Geometry check sheet. Reference: drawing and pictorial views, mm from the part's lowest x, y, z. A direction names the side the tool comes from. Coordinates: 2 decimals unless noted, no trailing zeros. Order: outer loops, then holes, each group sorted by start corner. A loop starts at its lowest first (then second) coordinate and runs counter-clockwise, first axis right, second up. Notation, with made-up numbers: M 29.5,50 L 59.5,50 A21 ccw 59.5,67 Z; hole C 48,-1 d7. An arc over 180 degrees is marked long. Return JSON: item names as keys, results as strings.
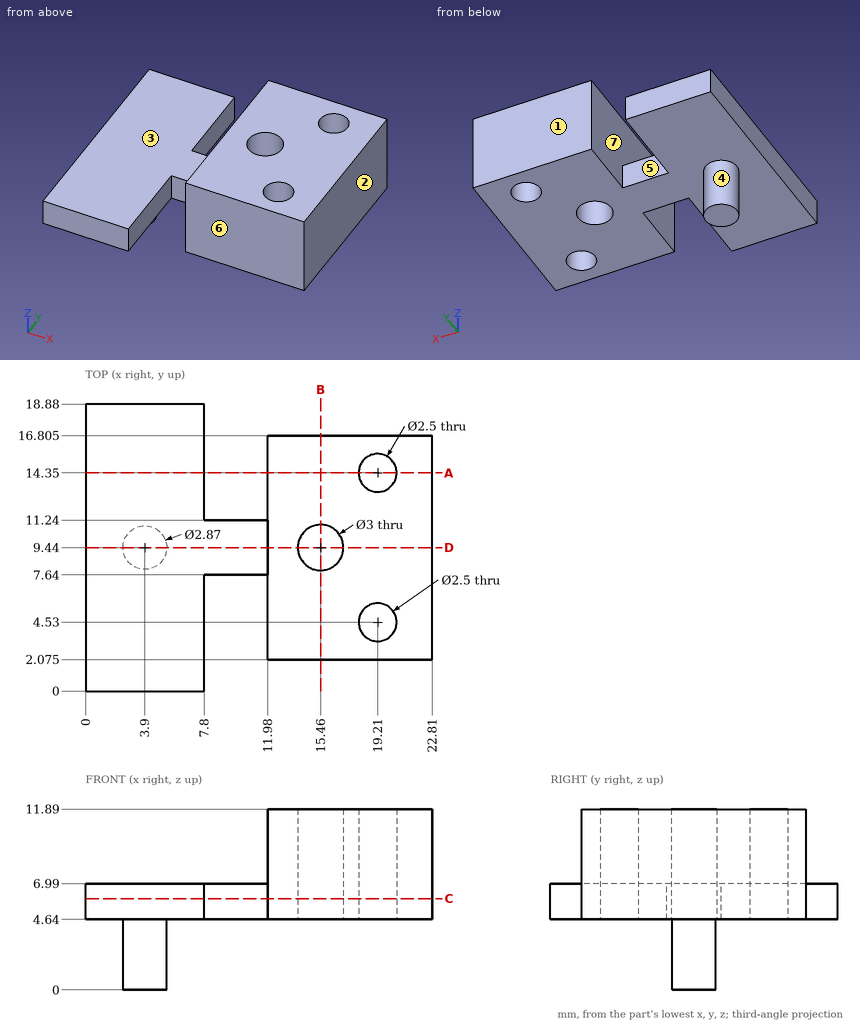
Q1. Go/stop test with flat-tipped pins: pin 1 (3 mm diameter, centred on x = 10, z = 5.5, fed in from -Y); pin 2 (6 mm diameter, centred on x = 16, z = 8.5, fed in from -Y) (3 decimals); pin 3 (9.5 mm diameter, centred on x = 15, y = 11.5, fed in from -Z). Record where each tip stops, or that it passes through.
Values:
{"pin 1": "y = 7.64", "pin 2": "y = 2.075", "pin 3": "z = 4.64"}
Q2. Cross-section at C-C, the plane z = 6. Record the boundary of the cut face in (x, y) (3 decimals), and give its area (3 significant figures).
Values:
{"outline": "M 0,0 L 7.8,0 L 7.8,7.64 L 11.98,7.64 L 11.98,2.075 L 22.81,2.075 L 22.81,16.805 L 11.98,16.805 L 11.98,11.24 L 7.8,11.24 L 7.8,18.88 L 0,18.88 Z; hole C 15.46,9.44 d3; hole C 19.21,4.53 d2.5; hole C 19.21,14.35 d2.5", "area": "305 mm^2"}
Q3. Cross-section at A-A, the plane y = 14.35. Record the boundary of the cut face in (x, z), and give its area (3 significant figures).
Values:
{"outline": "M 0,4.64 L 7.8,4.64 L 7.8,6.99 L 0,6.99 Z; M 11.98,4.64 L 17.96,4.64 L 17.96,11.89 L 11.98,11.89 Z; M 20.46,4.64 L 22.81,4.64 L 22.81,11.89 L 20.46,11.89 Z", "area": "78.7 mm^2"}
Q4. Cross-section at D-D, the plane y = 9.44. Record the boundary of the cut face in (x, z) (3 decimals), and give its area (3 significant figures).
Values:
{"outline": "M 0,4.64 L 2.465,4.64 L 2.465,0 L 5.335,0 L 5.335,4.64 L 13.96,4.64 L 13.96,11.89 L 11.98,11.89 L 11.98,6.99 L 0,6.99 Z; M 16.96,4.64 L 22.81,4.64 L 22.81,11.89 L 16.96,11.89 Z", "area": "98.2 mm^2"}
Q5. Tool access check on the marked faces 1, 2 and 3. Record the directions out of +Z, -Z, +X, -X, +Y, -Y that give a thin tool (end or side, any length) a straight path to the whole face; none if there is none.
Values:
{"face 1": "+Z, -Z, +X, +Y", "face 2": "+Z, -Z, +X, +Y, -Y", "face 3": "+Z, -X, +Y, -Y"}
Q6. Material ranges on line 1 along Y through (x, z) = (19.21, 7.25) (3 decimals); line 2 along Y through (x, z) = (15.46, 6.25) (3 decimals); line 3 along Z through (x, y) = (16, 3), recorded low to high.
Values:
{"line 1": "2.075 to 3.28, 5.78 to 13.1, 15.6 to 16.805", "line 2": "2.075 to 7.94, 10.94 to 16.805", "line 3": "4.64 to 11.89"}
Q7. Cross-section at B-B, the plane x = 15.46. Record the boundary of the cut face in (y, z) (3 decimals), and give its area (3 significant figures).
Values:
{"outline": "M 2.075,4.64 L 7.94,4.64 L 7.94,11.89 L 2.075,11.89 Z; M 10.94,4.64 L 16.805,4.64 L 16.805,11.89 L 10.94,11.89 Z", "area": "85.0 mm^2"}
Q8. Draft check along X on the marked faces 4, 5, 6 and 7. Enter one of: pulls with the +X half, pulls with the -X half, needs draft (parallel to the pull), parting line crosses it, or undercut.
Values:
{"face 4": "parting line crosses it", "face 5": "undercut", "face 6": "needs draft", "face 7": "undercut"}
